Could you check a few things on this model? Use its own coordinates, in mm. A direction names the side the tool comes from. Give positions to 0.01 mm unless a question says otherwise; leave off trailing zeros. Write each loop counter-clockwise with the first axis right and the second up, starting at its lowest first coordinate (ties: lowest second). Pieces come first, ordered by that corner, then holes. Notation, with made-up numbers: M 44.25,32.25 L 89.25,32.25 A18 cw 89.25,59.25 Z; hole C 56.5,-16 d6. An arc over 180 degrees is marked long. Use one line per item in the form item = value.
Autodesk Inventor part; units mm, degrees
ref_plane "YZ Plane" through (0, 0, 0) normal (1, 0, 0) x (0, 1, 0)
ref_plane "XZ Plane" through (0, 0, 0) normal (0, 1, 0) x (-1, 0, 0)
ref_plane "XY Plane" through (0, 0, 0) normal (0, 0, 1) x (1, 0, 0)
sketch "Sketch1" plane through (0, 0, 0) normal (1, 0, 0) x (0, 1, 0)
  circle A0 centre (0, 0) radius 3.25
  circle A1 centre (0, 0) radius 4.75
  line L0 (-4.75, 0) -> (-4.75, -20)
  line L1 (-4.75, 0) -> (-4.75, 20)
  line L2 (-4.75, 20) -> (-0.75, 20)
  line L3 (-0.75, 20) -> (-0.75, 4.6904)
  line L4 (-0.75, -4.6904) -> (-0.75, -20)
  line L5 (-4.75, -20) -> (-0.75, -20)
  line L6 (3.2538, 3.4605) -> (-0.75, 7.2252)
  line L7 (3.2538, -3.4605) -> (-0.75, -7.7187)
  dimension "d0" = 6.5
  dimension "d1" = 9.5
  dimension "d2" = 20
  dimension "d3" = 20
  dimension "d4" = 4
extrude "Extrusion1" add sketch "Sketch1" along normal blind 20
sketch "Sketch3" plane through (0, -0.75, 20) normal (0, 1, 0) x (1, 0, 0)
  line L0 (0, 0) -> (0, 40)
  line L1 (0, 0) -> (10, 0)
  line L2 (0, 0) -> (20, 0)
  line L3 (10, 0) -> (10, 6.5)
  line L4 (0, 40) -> (20, 40)
  line L5 (0, 40) -> (10, 40)
  line L6 (10, 40) -> (10, 33.5)
  circle A0 centre (10, 6.5) radius 2.5
  circle A1 centre (10, 33.5) radius 2.5
  point P0 (0, 20)
  dimension "d7" = 6.5
  dimension "d8" = 6.5
  dimension "d9" = 5
  dimension "d10" = 5
extrude "Extrusion2" cut sketch "Sketch3" against normal blind 20
fillet "Fillet1" radius 2 2 edges at (10, -0.75, 7.2252) (10, -0.75, -7.7187)
sketch "Sketch4" plane through (20, 0, 0) normal (1, 0, 0) x (0, 0, -1)
  circle A0 centre (0, 0) radius 3.25
extrude "Extrusion3" add sketch "Sketch4" against normal blind 10
sketch "Sketch5" plane through (0, -4.75, -20) normal (0, -1, 0) x (1, 0, 0)
  line L0 (0, 0) -> (20, 0)
  line L1 (20, 40) -> (20, 0)
  line L2 (0, 0) -> (20, 0)
  line L3 (20, 0) -> (20, 40)
  line L4 (20, 40) -> (0, 40)
  line L5 (0, 40) -> (0, 0)
  circle A0 centre (10, 6.5) radius 2.5
  circle A1 centre (10, 6.5) radius 2.5
  circle A2 centre (10, 33.5) radius 2.5
  circle A3 centre (10, 33.5) radius 2.5
  point P0 (0, 20)
extrude "Extrusion4" add sketch "Sketch5" along normal blind 9.75
sketch "Sketch6" plane through (0, -0.75, -20) normal (0, 1, 0) x (1, 0, 0)
  circle A0 centre (10, -6.5) radius 2.5
  circle A1 centre (10, -6.5) radius 7.5
  circle A2 centre (10, -33.5) radius 2.5
  circle A3 centre (10, -33.5) radius 7.5
  point P0 (0, -20)
  dimension "d18" = 15
  dimension "d19" = 15
extrude "Extrusion5" cut sketch "Sketch6" along normal blind 9.75
properties part number "linac_lower_ax_mount"
1) I want a section at B-B, the plane y = -9. Please give me the cut outline in (x, z).
Checked values:
outline = M 0,-20 L 20,-20 L 20,20 L 0,20 Z; hole C 10,-13.5 d5; hole C 10,13.5 d5
2) Thinking about a two-plate mould opening in Y: for faces 6 (the flat face through (9.86, 1.59, 5.024)), 7 (the flat face through (10, -8, -20)), 8 (the cylindrical face through (4.93, -2.579, 1.978)), which applies, released by +Y, released by -Y, zero draft, split by the parting line, or undercut?
Checked values:
face_6 = released by +Y
face_7 = zero draft
face_8 = undercut
3) If I drill on L1, parallel to Z at x = 10, y = -6.25; L2, parallel to Z at x = 7.75, y = -0.25; L3, parallel to Z at x = 11, y = -6, over which ranges is the centre line in solid material (lowest first)?
Checked values:
L1 = -20 to -16, -11 to 11, 16 to 20
L2 = -6.35 to -3.24, 3.24 to 6.35
L3 = -20 to -15.79, -11.21 to 11.21, 15.79 to 20
4) For pin 1 Ø10 at (x, z) = (3.5, -11) entering from +Y; pin 2 Ø4.5 at (x, z) = (10, -13.5) entering from +Y; pin 3 Ø4 at (x, z) = (6.5, 14.5) entering from +Y; pin 4 Ø6 at (y, z) = (0, 0) entering from -X, each with a flat end and sliding along its axis, tell me the tip position at first contact or that it passes through.
Checked values:
pin_1 = 0.87
pin_2 = through
pin_3 = -0.75
pin_4 = 10
5) I want a section at A-A, the plane z = 13.5. Please give me the cut outline in (x, y).
Checked values:
outline = M 0,-14.5 L 7.5,-14.5 L 7.5,-0.75 L 0,-0.75 Z; M 12.5,-14.5 L 20,-14.5 L 20,-0.75 L 12.5,-0.75 Z
6) For faces 1 (the flat face through (8, -0.75, -16)), 2 (the cylindrical face through (9.46, -7.53, 15.94)), 3 (the flat face through (10, 0, 0)), 4 (the cylindrical face through (17.33, -0.59, 7.31)), 5 (the cylindrical face through (10, 0, 6)), which set-ups out of +Z, -Z, +X, -X, +Y, -Y let a thin tool reach every point of the face, with its end or its side?
Checked values:
face_1 = -Z, +Y
face_2 = +Y, -Y
face_3 = -X
face_4 = +Z, +X, -X, +Y
face_5 = +Z, +Y
7) I want a section at D-D, the plane x = 13.5. Please give me the cut outline in (y, z).
Checked values:
outline = M -14.5,-20 L -0.75,-20 L -0.75,-6.87 L 0.05,-6.87 L 3.25,-3.46 A4.75 ccw 3.25,3.46 L -0.12,6.63 A2 cw -0.33,6.87 L -0.75,6.87 L -0.75,20 L -14.5,20 Z
8) I want a section at C-C, the plane z = 0. Please give me the cut outline in (x, y).
Checked values:
outline = M 0,-14.5 L 20,-14.5 L 20,4.75 L 0,4.75 L 0,3.25 L 10,3.25 L 10,-3.25 L 0,-3.25 Z
